from build123d import *

# Parameters (mm, degrees)
BOSS_EXTRUDE1_DEPTH      = 76
BOSS_EXTRUDE1_DEPTH_BACK = 76
SKETCH2_R                = 8
FILLET1_R                = 3
FILLET2_R                = 2
FILLET3_R                = 1
CUT_EXTRUDE2_DEPTH       = 155.090108397
CUT_EXTRUDE2_DEPTH_BACK  = 155.090108397
SKETCH7_R                = 3.5
SKETCH9_R                = 7
CUT_EXTRUDE3_DEPTH       = 8
CUT_EXTRUDE4_DEPTH       = 155.090108397
CUT_EXTRUDE4_DEPTH_BACK  = 155.090108397
SKETCH10_W               = 42
SKETCH10_H               = 59.343909382
SKETCH11_W               = 0.2
SKETCH11_H               = 2.5
BOSS_EXTRUDE2_DEPTH      = 0.2
FILLET4_R                = 0.1
CIRPATTERN1_COUNT        = 8
FILLET4_OF_CIRPATTERN1_R = 0.1
MIRROR2_START            = 118.5
MIRROR2_DEPTH            = 2.5
MIRROR2_START_2          = 129
MIRROR2_2_DEPTH          = 2.5
MIRROR2_START_3          = 87.545201898
MIRROR2_3_DEPTH          = 2.5
MIRROR2_START_4          = 98.045201898
MIRROR2_4_DEPTH          = 2.5
MIRROR2_START_5          = 1.5
MIRROR2_5_DEPTH          = 2.5
MIRROR2_START_6          = 12
MIRROR2_6_DEPTH          = 2.5
MIRROR2_START_7          = -89.231493399
MIRROR2_7_DEPTH          = 2.5
MIRROR2_START_8          = -78.731493399
MIRROR2_8_DEPTH          = 2.5


# Read off the part's stored shape, not the designer's step: Mirror2
with BuildPart() as part:
    # Sketch2 → Boss-Extrude1 (new, two sides: drawn at the far end of the back side and taken through both)
    with BuildSketch(Plane.XY.offset(-BOSS_EXTRUDE1_DEPTH_BACK)):
        with Locations((8, 125)):
            Circle(SKETCH2_R)
        with BuildLine():
            ThreePointArc((8, 117), (5.350470229, 117.451490744), (3, 118.755002002))
            Line((3, 118.755002002), (3, 117))
            Line((3, 117), (8, 117))
        make_face()
        with BuildLine():
            Line((0, 125), (0, 0))
            Line((0, 0), (-11, 0))
            Line((-11, 0), (-14.464101615, 6))
            Line((-14.464101615, 6), (-17.062177826, 4.5))
            Line((-17.062177826, 4.5), (-12.732050808, -3))
            Line((-12.732050808, -3), (3, -3))
            Line((3, -3), (3, 117))
            Line((3, 117), (3, 118.755002002))
            ThreePointArc((3, 118.755002002), (0.788897449, 121.535898385), (0, 125))
        make_face()
    extrude(amount=BOSS_EXTRUDE1_DEPTH + BOSS_EXTRUDE1_DEPTH_BACK)

    # Fillet1
    fillet1_edges = [part.edges().sort_by_distance(p)[0] for p in [
        (3, -3, 0),
        (-12.732050808, -3, 0),
    ]]
    fillet(fillet1_edges, radius=FILLET1_R)

    # Fillet2
    fillet2_edges = [part.edges().sort_by_distance(p)[0] for p in [
        (-11, 0, 0),
        (0, 0, 0),
    ]]
    fillet(fillet2_edges, radius=FILLET2_R)

    # Fillet3
    fillet3_edges = [part.edges().sort_by_distance(p)[0] for p in [
        (-17.062177826, 4.5, 0),
        (-14.464101615, 6, 0),
    ]]
    fillet(fillet3_edges, radius=FILLET3_R)

    # Sketch7 → Cut-Extrude2 (cut, two sides: drawn at the far end of the back side and taken through both)
    with BuildSketch(Plane.XY.offset(-CUT_EXTRUDE2_DEPTH_BACK)):
        with Locations((8, 125)):
            Circle(SKETCH7_R)
    extrude(amount=CUT_EXTRUDE2_DEPTH + CUT_EXTRUDE2_DEPTH_BACK, mode=Mode.SUBTRACT)

    # Sketch9 → Cut-Extrude3 (cut)
    with BuildSketch(Plane.XY.offset(76)):
        with Locations((8, 125)):
            Circle(SKETCH9_R)
    cut_extrude3 = extrude(amount=-CUT_EXTRUDE3_DEPTH, mode=Mode.SUBTRACT)

    # Mirror1: Cut-Extrude3 across plane
    add(cut_extrude3.mirror(Plane.XY), mode=Mode.SUBTRACT)

    # Sketch10 → Cut-Extrude4 (cut, two sides: drawn at the far end of the back side and taken through both)
    with BuildSketch(Plane(origin=(0, 0, 0), x_dir=(0, 0, -1), z_dir=(1, 0, 0)).offset(-CUT_EXTRUDE4_DEPTH_BACK)):
        with Locations((0, 144.671954691)):
            Rectangle(SKETCH10_W, SKETCH10_H)
    extrude(amount=CUT_EXTRUDE4_DEPTH + CUT_EXTRUDE4_DEPTH_BACK, mode=Mode.SUBTRACT)

    # Sketch11 → Boss-Extrude2 (add)
    with BuildSketch(Plane.XY.offset(-21)):
        with Locations((8, 130.25)):
            Rectangle(SKETCH11_W, SKETCH11_H)
    boss_extrude2 = extrude(amount=BOSS_EXTRUDE2_DEPTH)

    # Fillet4
    fillet4_edges = [part.edges().sort_by_distance(p)[0] for p in [
        (8.1, 130.25, -20.8),
        (7.9, 130.25, -20.8),
    ]]
    fillet(fillet4_edges, radius=FILLET4_R - 0.0001)  # a hair under: the kernel refuses the full size

    # CirPattern1: Boss-Extrude2 ×8 about axis
    cirpattern1_axis = Axis((8, 125, 0), (0, 0, 1))
    for i in range(1, CIRPATTERN1_COUNT):
        add(boss_extrude2.rotate(cirpattern1_axis, i * 360 / CIRPATTERN1_COUNT))

    # Fillet4 of CirPattern1
    fillet4_of_cirpattern1_edges = [part.edges().sort_by_distance(p)[0] for p in [
        (4.358400077, 128.783021279, -20.8),
        (4.216978721, 128.641599923, -20.8),
        (2.75, 125.1, -20.8),
        (2.75, 124.9, -20.8),
        (4.216978721, 121.358400077, -20.8),
        (4.358400077, 121.216978721, -20.8),
        (7.9, 119.75, -20.8),
        (8.1, 119.75, -20.8),
        (11.641599923, 121.216978721, -20.8),
        (11.783021279, 121.358400077, -20.8),
        (13.25, 124.9, -20.8),
        (13.25, 125.1, -20.8),
        (11.783021279, 128.641599923, -20.8),
        (11.641599923, 128.783021279, -20.8),
    ]]
    fillet(fillet4_of_cirpattern1_edges, radius=FILLET4_OF_CIRPATTERN1_R - 0.0001)  # a hair under: the kernel refuses the full size

    # Mirror2 outline → Mirror2 (add)
    with BuildSketch(Plane(origin=(0, 0, 0), x_dir=(1, 0, 0), z_dir=(0, 1, 0)).offset(MIRROR2_START)):
        with BuildLine():
            Line((7.9, -21), (8.1, -21))
            Line((8.1, -21), (8.1, -20.9))
            ThreePointArc((8.1, -20.9), (8.070710678, -20.829289322), (8, -20.8))
            ThreePointArc((8, -20.8), (7.929289322, -20.829289322), (7.9, -20.9))
            Line((7.9, -20.9), (7.9, -21))
        make_face()
    extrude(amount=MIRROR2_DEPTH)

    # Mirror2 2 outline → Mirror2 2 (add)
    with BuildSketch(Plane(origin=(0, 0, 0), x_dir=(1, 0, 0), z_dir=(0, 1, 0)).offset(MIRROR2_START_2)):
        with BuildLine():
            Line((7.9, -21), (8.1, -21))
            Line((8.1, -21), (8.1, -20.9))
            ThreePointArc((8.1, -20.9), (8.070710678, -20.829289322), (8, -20.8))
            ThreePointArc((8, -20.8), (7.929289322, -20.829289322), (7.9, -20.9))
            Line((7.9, -20.9), (7.9, -21))
        make_face()
    extrude(amount=MIRROR2_2_DEPTH)

    # Mirror2 3 outline → Mirror2 3 (add)
    with BuildSketch(Plane(origin=(0, 0, 0), x_dir=(0.7071067811865471, -0.707106781186548, 0), z_dir=(0.707106781186548, 0.707106781186547, 0)).offset(MIRROR2_START_3)):
        with BuildLine():
            Line((-82.831493399, -21), (-82.631493399, -21))
            Line((-82.631493399, -21), (-82.631493399, -20.9))
            ThreePointArc((-82.631493399, -20.9), (-82.660782721, -20.829289322), (-82.731493399, -20.8))
            ThreePointArc((-82.731493399, -20.8), (-82.802204077, -20.829289322), (-82.831493399, -20.9))
            Line((-82.831493399, -20.9), (-82.831493399, -21))
        make_face()
    extrude(amount=MIRROR2_3_DEPTH)

    # Mirror2 4 outline → Mirror2 4 (add)
    with BuildSketch(Plane(origin=(0, 0, 0), x_dir=(0.7071067811865471, -0.707106781186548, 0), z_dir=(0.707106781186548, 0.707106781186547, 0)).offset(MIRROR2_START_4)):
        with BuildLine():
            Line((-82.831493399, -21), (-82.631493399, -21))
            Line((-82.631493399, -21), (-82.631493399, -20.9))
            ThreePointArc((-82.631493399, -20.9), (-82.660782721, -20.829289322), (-82.731493399, -20.8))
            ThreePointArc((-82.731493399, -20.8), (-82.802204077, -20.829289322), (-82.831493399, -20.9))
            Line((-82.831493399, -20.9), (-82.831493399, -21))
        make_face()
    extrude(amount=MIRROR2_4_DEPTH)

    # Mirror2 5 outline → Mirror2 5 (add)
    with BuildSketch(Plane.YZ.offset(MIRROR2_START_5)):
        with BuildLine():
            Line((125.1, 21), (124.9, 21))
            Line((124.9, 21), (124.9, 20.9))
            ThreePointArc((124.9, 20.9), (124.929289322, 20.829289322), (125, 20.8))
            ThreePointArc((125, 20.8), (125.070710678, 20.829289322), (125.1, 20.9))
            Line((125.1, 20.9), (125.1, 21))
        make_face()
    extrude(amount=MIRROR2_5_DEPTH)

    # Mirror2 6 outline → Mirror2 6 (add)
    with BuildSketch(Plane.YZ.offset(MIRROR2_START_6)):
        with BuildLine():
            Line((125.1, 21), (124.9, 21))
            Line((124.9, 21), (124.9, 20.9))
            ThreePointArc((124.9, 20.9), (124.929289322, 20.829289322), (125, 20.8))
            ThreePointArc((125, 20.8), (125.070710678, 20.829289322), (125.1, 20.9))
            Line((125.1, 20.9), (125.1, 21))
        make_face()
    extrude(amount=MIRROR2_6_DEPTH)

    # Mirror2 7 outline → Mirror2 7 (add)
    with BuildSketch(Plane(origin=(0, 0, 0), x_dir=(0.7071067811865509, 0.707106781186544, 0), z_dir=(0.707106781186544, -0.707106781186551, 0)).offset(MIRROR2_START_7)):
        with BuildLine():
            Line((94.145201898, 21), (93.945201898, 21))
            Line((93.945201898, 21), (93.945201898, 20.9))
            ThreePointArc((93.945201898, 20.9), (93.97449122, 20.829289322), (94.045201898, 20.8))
            ThreePointArc((94.045201898, 20.8), (94.115912576, 20.829289322), (94.145201898, 20.9))
            Line((94.145201898, 20.9), (94.145201898, 21))
        make_face()
    extrude(amount=MIRROR2_7_DEPTH)

    # Mirror2 8 outline → Mirror2 8 (add)
    with BuildSketch(Plane(origin=(0, 0, 0), x_dir=(0.7071067811865509, 0.707106781186544, 0), z_dir=(0.707106781186544, -0.707106781186551, 0)).offset(MIRROR2_START_8)):
        with BuildLine():
            Line((94.145201898, 21), (93.945201898, 21))
            Line((93.945201898, 21), (93.945201898, 20.9))
            ThreePointArc((93.945201898, 20.9), (93.97449122, 20.829289322), (94.045201898, 20.8))
            ThreePointArc((94.045201898, 20.8), (94.115912576, 20.829289322), (94.145201898, 20.9))
            Line((94.145201898, 20.9), (94.145201898, 21))
        make_face()
    extrude(amount=MIRROR2_8_DEPTH)


solid = part.part
The listing builds one solid part. Answer for the finished solid, in the listing's coordinates (mm). A direction names the side the tool comes from. Coordinates: 2 decimals unless noted, no trailing zeros. Loops run counter-clockwise (first coordinate to the right, second up) from the corner with the lowest first, then second, coordinate; pieces in that order, holes last. Notation, with made-up numbers: (-7.75, -11.5) -> (47.25, -11.5) arc R19 cw to (47.25, -0.5) -> close; hole circle Ø7 at (-3, 74.5). An arc over 180 degrees is marked (long way). Answer in a Markdown table with one row per item. Add a question column.
1. The part is cut by section D-D, the plane y = 83. Write down the section's boundary in (x, z).
2. The part is cut by section A-A, the plane z = -4. Write down the section's boundary in (x, y), then the cut area to 3 significant figures.
3. For faces 1 (the cylindrical face through (11.763, 130.902, 72.056)), 2 (the flat face through (5, 117, 48)), 3 (the flat face through (11, 122, -68)), determine the directions among +Z, -Z, +X, -X, +Y, -Y from which every point of the face is accessible in a straight line to the end or side of a thin tool.
4. Determine the mould class of faces 4 (the flat face through (6.11, 121.87, 21)), 5 (the cylindrical face through (13.84, 130.47, -48.89)), 6 (the flat face through (3, 58, -1)) for opening direction Y: +Y half, -Y half, draft (parallel to the pull), parting line (faces both ways), or undercut.
5. Flat-ended cylindrical pins translate along their axes: P1, Ø9, axis at x = 8, y = 125, coming from the +Z side; P2, Ø4, axis at x = 5, y = 126, coming from the -Z side; P3, Ø4, axis at x = -2.5, y = 110, coming from the -Z side; P4, Ø3, axis at x = -8, z = 47, coming from the +Y side. Find the tip coordinate at first contact, or state that the pin passes through.
6. The part is cut by section C-C, the plane x = -7.5. Write down the section's boundary in (y, z), then the cut area to 3 significant figures.
7. The part is cut by section B-B, the plane z = 60. Write down the section's boundary in (x, y), then the cut area to 3 significant figures.
8. Consider line 1 (Y direction, x = 8, z = -45); line 2 (X direction, y = 125, z = 38.5); line 3 (Y direction, x = 8, z = -73.25). Determine where each line is inside the solid, lowest interval first. Write a range as [from, to].
Answer below:
| question | item | result |
|---|---|---|
| 1 | outline | (0, -76) -> (3, -76) -> (3, 76) -> (0, 76) -> close |
| 2 | outline | (-16.56, 3.63) -> (-13.6, -1.5) arc R3 ccw to (-11, -3) -> (0, -3) arc R3 ccw to (3, 0) -> (3, 115) -> (0, 115) -> (0, 2) arc R2 cw to (-2, 0) -> (-9.85, 0) arc R2 cw to (-11.58, 1) -> (-13.96, 5.13) arc R1 ccw to (-15.33, 5.5) -> (-16.2, 5) arc R1 ccw to start |
| 2 | area | 411 mm2 |
| 3 | face 1 | +Z |
| 3 | face 2 | +Z, -Z, +X, -Y |
| 3 | face 3 | -Z |
| 4 | face 4 | undercut |
| 4 | face 5 | parting line |
| 4 | face 6 | draft |
| 5 | P1 | z = 68 |
| 5 | P2 | z = -68 |
| 5 | P3 | through |
| 5 | P4 | y = 0 |
| 6 | outline | (-3, -76) -> (0, -76) -> (0, 76) -> (-3, 76) -> close |
| 6 | area | 456 mm2 |
| 7 | outline | (-16.56, 3.63) -> (-13.6, -1.5) arc R3 ccw to (-11, -3) -> (0, -3) arc R3 ccw to (3, 0) -> (3, 117) -> (8, 117) arc R8 ccw (long way) to (0, 125) -> (0, 2) arc R2 cw to (-2, 0) -> (-9.85, 0) arc R2 cw to (-11.58, 1) -> (-13.96, 5.13) arc R1 ccw to (-15.33, 5.5) -> (-16.2, 5) arc R1 ccw to start; hole circle Ø7 at (8, 125) |
| 7 | area | 594 mm2 |
| 8 | line 1 | [117, 121.5], [128.5, 133] |
| 8 | line 2 | [0, 4.5], [11.5, 16] |
| 8 | line 3 | [117, 118], [132, 133] |
